The model under review builds one solid part; all positions refer to its coordinate system, in mm. A direction names the side the tool comes from. Round coordinates to 2 decimals unless told otherwise and drop trailing zeros. Loops run counter-clockwise (first coordinate to the right, second up) from the corner with the lowest first, then second, coordinate; pieces in that order, holes last. Notation, with made-up numbers: M 64.25,35.5 L 68.25,35.5 A24 ccw 68.25,64.5 Z; hole C 2,7.25 d3. An arc over 180 degrees is marked long. Return JSON: item names as keys, results as strings. Group by question number.
Q1. Consider section C-C (z = 19). State the section outline as (x, y) points, and give its area (3 significant figures).
Q2. For faces 5 (the face through (24, -7, 12)), 6 (the face through (24, -7, 24)), 7 (the face through (46.912, -1.426, 23.179)), 8 (the face through (25, -7, 11)), 9 (the face through (24.3, 0, 7.5)), list the 3-axis set-ups (+Z, -Z, +X, -X, +Y, -Y) from which the entire face can be reached by the end or side of a thin tool; tool diameter is ignored.
Q3. Consider section B-B (y = -7.5). State the section outline as (x, z) points, and give its area (3 significant figures).
Q4. To check wall thickness, follow line 1 along Z through (x, y) = (0, -8.5); line 2 along X through (y, z) = (-11.75, -0.5) (3 decimals); line 3 along X through (y, z) = (-13.25, 9). State the ranges of each line that lie inside material, in increasing order.
Q5. Draft analysis for pull direction Z (two halves, no side actions). For faces 1 (the face through (37, -7, 22.629)), 2 (the face through (37, -7, 23.715)), 3 (the face through (25, -7, 25)), 4 (the face through (24.3, -15, 7.5)), state which applies: pulls with the +Z half, pulls with the -Z half, needs draft (parallel to the pull), parting line crosses it, or undercut.
Q6. Consider section A-A (x = 32). State the section outline as (y, z) points, and give its area (3 significant figures).
Q7. Consider section D-D (y = -3.5). State the section outline as (x, z) points, and give its area (3 significant figures).
Q8. Clearance check with flat-ended pins moving along their axes: pin 1 Ø4.5 at (y, z) = (-9, 11.5) entering from -X; pin 2 Ø8 at (y, z) = (-3.5, -17.5) entering from +X; pin 3 Ø8 at (y, z) = (-4.5, -8.5) entering from +X. State where each tip first meets the part, or that it passes through.
from build123d import *

# Parameters (mm, degrees)
F1_DEPTH = 15
F2_R     = 2
F3_DEPTH = 25


with BuildPart() as f1:
    # F0 (on Front) → F1 (new body)
    with BuildSketch(Plane.XZ):
        with BuildLine():
            Line((48.415434, 25), (0, 25))
            ThreePointArc((0, 25), (-17.67767, -17.67767), (25, 0))
            Line((25, 0), (25, 21.628764))
            ThreePointArc((25, 21.628764), (25.292893, 22.33587), (26, 22.628764))
            Line((26, 22.628764), (48.415434, 22.628764))
            Line((48.415434, 22.628764), (48.415434, 23.714876))
            Line((48.415434, 23.714876), (25, 23.714876))
            ThreePointArc((25, 23.714876), (24.292893, 23.421983), (24, 22.714876))
            Line((24, 22.714876), (24, 7))
            Line((24, 7), (24, 0))
            ThreePointArc((24, 0), (-16.970563, -16.970563), (0, 24))
            Line((0, 24), (7, 24))
            Line((7, 24), (48.415434, 24))
            Line((48.415434, 24), (48.415434, 25))
        make_face()
    extrude(amount=F1_DEPTH)

    # F2 (on face) → F3 (cut)
    with BuildSketch(Plane.XY.offset(25)):
        with BuildLine():
            Line((48.415434, 0), (43.415434, 0))
            ThreePointArc((43.415434, 0), (46.950968, -1.464466), (48.415434, -5))
            Line((48.415434, -5), (48.415434, 0))
        make_face()
        with BuildLine():
            Line((48.415434, -15), (48.415434, -10))
            ThreePointArc((48.415434, -10), (46.950968, -13.535534), (43.415434, -15))
            Line((43.415434, -15), (48.415434, -15))
        make_face()
        with Locations((43.415434, -7.5)):
            Circle(F2_R)
    extrude(amount=-F3_DEPTH, mode=Mode.SUBTRACT)


solid = f1.part
Values:
{
 "1": {"outline": "M -16.25,-15 L -14.66,-15 L -14.66,0 L -16.25,0 Z; M 24,-15 L 25,-15 L 25,0 L 24,0 Z", "area": "38.8 mm2"},
 "2": {"face 5": "+Y, -Y", "face 6": "+X, +Y, -Y", "face 7": "+Z, -Z, +X, +Y", "face 8": "-Z, +X, +Y, -Y", "face 9": "+Z, -Z, +X, -X, +Y"},
 "3": {"outline": "M 0,24 L 41.42,24 L 41.42,25 L 0,25 A25 ccw long 25,0 L 25,21.63 A1 cw 26,22.63 L 41.42,22.63 L 41.42,23.71 L 25,23.71 A1 ccw 24,22.71 L 24,0 A24 cw long Z; M 45.42,22.63 L 48.42,22.63 L 48.42,23.71 L 45.42,23.71 Z; M 45.42,24 L 48.42,24 L 48.42,25 L 45.42,25 Z", "area": "205 mm2"},
 "4": {"line 1": "z = -25 to -24, 24 to 25", "line 2": "x = -24.995 to -23.995, 23.995 to 24.995", "line 3": "x = -23.32 to -22.25, 24 to 25"},
 "5": {"face 1": "pulls with the -Z half", "face 2": "undercut", "face 3": "pulls with the +Z half", "face 4": "needs draft"},
 "6": {"outline": "M -15,22.63 L 0,22.63 L 0,23.71 L -15,23.71 Z; M -15,24 L 0,24 L 0,25 L -15,25 Z", "area": "31.3 mm2"},
 "7": {"outline": "M 0,24 L 48.19,24 L 48.19,25 L 0,25 A25 ccw long 25,0 L 25,21.63 A1 cw 26,22.63 L 48.19,22.63 L 48.19,23.71 L 25,23.71 A1 ccw 24,22.71 L 24,0 A24 cw long Z", "area": "213 mm2"},
 "8": {"pin 1": "stops at x = -23.23", "pin 2": "stops at x = 21.04", "pin 3": "stops at x = 24.59"}
}
